Verification items for the finished model (mm, model axes). Round coordinates to 2 decimals unless told otherwise and drop trailing zeros. Write each loop counter-clockwise with the first axis right and the second up, starting at its lowest first coordinate (ties: lowest second). Pieces come first, ordered by that corner, then holes. Notation, with made-up numbers: M 53,-10.5 L 98,-10.5 A23 cw 98,12.5 Z; hole C 10.5,52 d7. An arc over 180 degrees is marked long. One line per question, with ' | ' between items. Start each with the question number.
Q1. Thickness scan on line 1 along Y through (x, z) = (-91, 2.45); line 2 along X through (y, z) = (84, 0.7); line 3 along Y through (x, z) = (-38, 1.65). Record the ranges inside material, lowest first. Write a range as from..to.
Q2. Cross-section at B-B (z = 2.6). State how many separate pieces and enclosed holes the cut face has, then the cut area to 3 significant figures.
Q3. Cross-section at A-A (y = -96). Record the boundary of the cut face in (x, z) (3 decimals), then the cut area to 3 significant figures.
from build123d import *

# Parameters (mm, degrees)
SKETCH1_W           = 441.979400076
SKETCH1_H           = 305.81676
BOSS_EXTRUDE1_DEPTH = 3.175
CUT_EXTRUDE1_DEPTH  = 271.654843319
CUT_EXTRUDE2_DEPTH  = 271.654843319
LPATTERN1_COUNT     = 3
LPATTERN1_PITCH     = 181.613999992
LPATTERN2_COUNT     = 2
LPATTERN2_PITCH     = 181.613999992
CUT_EXTRUDE3_DEPTH  = 271.654843319
FILLET1_R           = 2


with BuildPart() as part:
    # Sketch1 → Boss-Extrude1 (new body)
    with BuildSketch(Plane.XY):
        with Locations((0, -3.32067)):
            Rectangle(SKETCH1_W, SKETCH1_H)
    extrude(amount=BOSS_EXTRUDE1_DEPTH)

    # Sketch2 → Cut-Extrude1 (cut, through all)
    with BuildSketch(Plane.XY.offset(3.175)):
        with BuildLine():
            Line((-185.746625, -116.8), (-166.696625, -116.8))
            ThreePointArc((-166.696625, -116.8), (-164.45156097, -115.87006403), (-163.521625, -113.625))
            Line((-163.521625, -113.625), (-163.521625, -81.875))
            ThreePointArc((-163.521625, -81.875), (-164.45156097, -79.62993597), (-166.696625, -78.7))
            Line((-166.696625, -78.7), (-185.746625, -78.7))
            ThreePointArc((-185.746625, -78.7), (-187.99168903, -79.62993597), (-188.921625, -81.875))
            Line((-188.921625, -81.875), (-188.921625, -113.625))
            ThreePointArc((-188.921625, -113.625), (-187.99168903, -115.87006403), (-185.746625, -116.8))
        make_face()
        with BuildLine():
            Line((-185.746625, 78.7), (-166.696625, 78.7))
            ThreePointArc((-166.696625, 78.7), (-164.45156097, 79.62993597), (-163.521625, 81.875))
            Line((-163.521625, 81.875), (-163.521625, 113.625))
            ThreePointArc((-163.521625, 113.625), (-164.45156097, 115.87006403), (-166.696625, 116.8))
            Line((-166.696625, 116.8), (-185.746625, 116.8))
            ThreePointArc((-185.746625, 116.8), (-187.99168903, 115.87006403), (-188.921625, 113.625))
            Line((-188.921625, 113.625), (-188.921625, 81.875))
            ThreePointArc((-188.921625, 81.875), (-187.99168903, 79.62993597), (-185.746625, 78.7))
        make_face()
    cut_extrude1 = extrude(amount=-CUT_EXTRUDE1_DEPTH, mode=Mode.SUBTRACT)

    # Sketch3 → Cut-Extrude2 (cut, through all)
    with BuildSketch(Plane.XY.offset(3.175)):
        with BuildLine():
            Line((-108.906375, -81.875), (-108.906375, -113.625))
            ThreePointArc((-108.906375, -113.625), (-107.97643903, -115.87006403), (-105.731375, -116.8))
            Line((-105.731375, -116.8), (-86.681375, -116.8))
            ThreePointArc((-86.681375, -116.8), (-84.43631097, -115.87006403), (-83.506375, -113.625))
            Line((-83.506375, -113.625), (-83.506375, -81.875))
            ThreePointArc((-83.506375, -81.875), (-84.43631097, -79.62993597), (-86.681375, -78.7))
            Line((-86.681375, -78.7), (-105.731375, -78.7))
            ThreePointArc((-105.731375, -78.7), (-107.97643903, -79.62993597), (-108.906375, -81.875))
        make_face()
        with BuildLine():
            Line((-83.506375, 81.875), (-83.506375, 113.625))
            ThreePointArc((-83.506375, 113.625), (-84.43631097, 115.87006403), (-86.681375, 116.8))
            Line((-86.681375, 116.8), (-105.731375, 116.8))
            ThreePointArc((-105.731375, 116.8), (-107.97643903, 115.87006403), (-108.906375, 113.625))
            Line((-108.906375, 113.625), (-108.906375, 81.875))
            ThreePointArc((-108.906375, 81.875), (-107.97643903, 79.62993597), (-105.731375, 78.7))
            Line((-105.731375, 78.7), (-86.681375, 78.7))
            ThreePointArc((-86.681375, 78.7), (-84.43631097, 79.62993597), (-83.506375, 81.875))
        make_face()
    cut_extrude2 = extrude(amount=-CUT_EXTRUDE2_DEPTH, mode=Mode.SUBTRACT)

    # LPattern1: Cut-Extrude1 ×3
    with Locations(*[(i * LPATTERN1_PITCH, 0, 0) for i in range(1, LPATTERN1_COUNT)]):
        add(cut_extrude1, mode=Mode.SUBTRACT)

    # LPattern2: Cut-Extrude2 ×2
    with Locations(*[(i * LPATTERN2_PITCH, 0, 0) for i in range(1, LPATTERN2_COUNT)]):
        add(cut_extrude2, mode=Mode.SUBTRACT)

    # Sketch6 → Cut-Extrude3 (cut, through all)
    with BuildSketch(Plane.XY.offset(3.175)):
        with BuildLine():
            Line((-77.407000004, 92.08771), (-13.407000004, 92.08771))
            Line((-13.407000004, 92.08771), (-13.407000004, 126.58771))
            Line((-13.407000004, 126.58771), (-6.407000004, 126.58771))
            ThreePointArc((-6.407000004, 126.58771), (-3.578572879, 127.759282875), (-2.407000004, 130.58771))
            Line((-2.407000004, 130.58771), (-2.407000004, 137.58771))
            ThreePointArc((-2.407000004, 137.58771), (-3.578572879, 140.416137125), (-6.407000004, 141.58771))
            Line((-6.407000004, 141.58771), (-13.407000004, 141.58771))
            Line((-13.407000004, 141.58771), (-13.407000004, 149.58771))
            Line((-13.407000004, 149.58771), (-77.407000004, 149.58771))
            Line((-77.407000004, 149.58771), (-77.407000004, 141.58771))
            Line((-77.407000004, 141.58771), (-84.407000004, 141.58771))
            ThreePointArc((-84.407000004, 141.58771), (-87.235427129, 140.416137125), (-88.407000004, 137.58771))
            Line((-88.407000004, 137.58771), (-88.407000004, 130.58771))
            ThreePointArc((-88.407000004, 130.58771), (-87.235427129, 127.759282875), (-84.407000004, 126.58771))
            Line((-84.407000004, 126.58771), (-77.407000004, 126.58771))
            Line((-77.407000004, 126.58771), (-77.407000004, 92.08771))
        make_face()
    extrude(amount=-CUT_EXTRUDE3_DEPTH, mode=Mode.SUBTRACT)

    # Fillet1
    fillet1_edges = [part.edges().sort_by_distance(p)[0] for p in [
        (-77.407000004, 141.58771, 1.5875),
        (-77.407000004, 149.58771, 1.5875),
        (-13.407000004, 149.58771, 1.5875),
        (-13.407000004, 141.58771, 1.5875),
        (-13.407000004, 126.58771, 1.5875),
        (-13.407000004, 92.08771, 1.5875),
        (-77.407000004, 92.08771, 1.5875),
        (-77.407000004, 126.58771, 1.5875),
        (220.989700038, -156.22905, 1.5875),
        (-220.989700038, -156.22905, 1.5875),
        (-220.989700038, 149.58771, 1.5875),
        (220.989700038, 149.58771, 1.5875),
    ]]
    fillet(fillet1_edges, radius=FILLET1_R)


solid = part.part
Determined:
1) line 1: y = -156.23..-116.8, -78.7..78.7, 116.8..149.59 | line 2: x = -220.99..-188.92, -163.52..-108.91, -83.51..-7.31, 18.09..72.71, 98.11..174.31, 199.71..220.99 | line 3: y = -156.23..92.09
2) separate pieces: 1 | enclosed holes: 10 | area: 122,000 mm²
3) outline: M -220.99,0 L -188.922,0 L -188.922,3.175 L -220.99,3.175 Z; M -163.522,0 L -108.906,0 L -108.906,3.175 L -163.522,3.175 Z; M -83.506,0 L -7.308,0 L -7.308,3.175 L -83.506,3.175 Z; M 18.092,0 L 72.708,0 L 72.708,3.175 L 18.092,3.175 Z; M 98.108,0 L 174.306,0 L 174.306,3.175 L 98.108,3.175 Z; M 199.706,0 L 220.99,0 L 220.99,3.175 L 199.706,3.175 Z | area: 1,000 mm²
